For this review, take the finished solid that the model builds, in its own axes (mm). A direction names the side the tool comes from. Round coordinates to 2 decimals unless told otherwise and drop trailing zeros. Write each loop counter-clockwise with the first axis right and the second up, starting at its lowest first coordinate (ties: lowest second). Pieces come first, ordered by that corner, then holes. Notation, with made-up numbers: (25.5, 38.5) -> (32.5, 38.5) arc R25 cw to (32.5, 61.5) -> close; hole circle Ø7 at (-30, -12). An arc over 180 degrees is marked (long way). Answer in a Markdown table with one row per item.
from build123d import *

# Parameters (mm, degrees)
SKETCH_1_W                         = 26.8
SKETCH_1_H                         = 10.5
EXTRUDE_1_DEPTH                    = 8.6
CUT_EXTRUDE_1_DEPTH                = 7
EXTRUDE_START                      = -5
SKETCH_3_W                         = 1
SKETCH_3_H                         = 1
EXTRUDE_2_DEPTH                    = 8.6
CHAMFER_1_SIZE                     = 0.3
SKETCH_4_W                         = 1
SKETCH_4_H                         = 1
EXTRUDE_3_DEPTH                    = 5
PATTERN_LINEAR_1_COUNT             = 7
PATTERN_LINEAR_1_PITCH             = 3.5
CHAMFER_1_OF_PATTERN_LINEAR_1_SIZE = 0.3


with BuildPart() as part:
    # Эскиз1 → Бобышка-Вытянуть1 (new body)
    with BuildSketch(Plane.XY):
        with Locations((0, 5.25)):
            Rectangle(SKETCH_1_W, SKETCH_1_H)
    extrude(amount=EXTRUDE_1_DEPTH)

    # Эскиз2 → Вырез-Вытянуть1 (cut)
    with BuildSketch(Plane.XZ):
        Polygon((-12.4, 6.6), (12.4, 6.6), (12.4, 0.2), (10.2, 0.2), (10.2, 1.8), (-8.6, 1.8), (-8.6, 0.2), (-10.8, 0.2), (-10.8, 1.8), (-12.4, 1.8), align=None)
    extrude(amount=-CUT_EXTRUDE_1_DEPTH, mode=Mode.SUBTRACT)

    # Эскиз3 → Бобышка-Вытянуть2 (add)
    with BuildSketch(Plane(origin=(0, 0, 0), x_dir=(-1, 0, 0), z_dir=(0, 0, -1)).offset(EXTRUDE_START)):
        with Locations((10.5, 9.5)):
            Rectangle(SKETCH_3_W, SKETCH_3_H)
    extrude_2 = extrude(amount=EXTRUDE_2_DEPTH)

    # Фаска1
    chamfer_1_edges = [part.edges().sort_by_distance(p)[0] for p in [
        (-10, 9.5, -3.6),
        (-10.5, 9, -3.6),
        (-11, 9.5, -3.6),
        (-10.5, 10, -3.6),
    ]]
    chamfer(chamfer_1_edges, length=CHAMFER_1_SIZE)

    # Эскиз4 → Бобышка-Вытянуть3 (add)
    with BuildSketch(Plane.XZ.offset(-7)):
        with Locations((-10.5, 4.35)):
            Rectangle(SKETCH_4_W, SKETCH_4_H)
    extrude_3 = extrude(amount=EXTRUDE_3_DEPTH)

    # Линейный массив1: Бобышка-Вытянуть2, Бобышка-Вытянуть3 ×7
    with Locations(*[(i * PATTERN_LINEAR_1_PITCH, 0, 0) for i in range(1, PATTERN_LINEAR_1_COUNT)]):
        add(extrude_2)
        add(extrude_3)

    # Фаска1 of Линейный массив1
    chamfer_1_of_pattern_linear_1_edges = [part.edges().sort_by_distance(p)[0] for p in [
        (-6.5, 9.5, -3.6),
        (-7, 9, -3.6),
        (-7.5, 9.5, -3.6),
        (-7, 10, -3.6),
        (-3, 9.5, -3.6),
        (-3.5, 9, -3.6),
        (-4, 9.5, -3.6),
        (-3.5, 10, -3.6),
        (0.5, 9.5, -3.6),
        (0, 9, -3.6),
        (-0.5, 9.5, -3.6),
        (0, 10, -3.6),
        (4, 9.5, -3.6),
        (3.5, 9, -3.6),
        (3, 9.5, -3.6),
        (3.5, 10, -3.6),
        (7.5, 9.5, -3.6),
        (7, 9, -3.6),
        (6.5, 9.5, -3.6),
        (7, 10, -3.6),
        (11, 9.5, -3.6),
        (10.5, 9, -3.6),
        (10, 9.5, -3.6),
        (10.5, 10, -3.6),
    ]]
    chamfer(chamfer_1_of_pattern_linear_1_edges, length=CHAMFER_1_OF_PATTERN_LINEAR_1_SIZE)


solid = part.part
1) For line 1 (Z direction, x = 10.5, y = 6.75); line 2 (Z direction, x = -5.5, y = 2); line 3 (X direction, y = 4.5, z = 5.5), list the stretches that pass through material, from the lowest coordinate up. Write a range as [from, to].
Solved:
| item | result |
|---|---|
| line 1 | [0, 0.2], [3.85, 4.85], [6.6, 8.6] |
| line 2 | [0, 1.8], [6.6, 8.6] |
| line 3 | [-13.4, -12.4], [12.4, 13.4] |
2) Mouldability with a two-part tool opening along X and no side actions: class faces 1 (the flat face through (10.5, 10, -1.6)), 2 (the flat face through (-7, 5, 3.85)), 3 (the flat face through (11, 9.5, -1.6)), 4 (the flat face through (0, 7, 3)) as pulls with the +X half, pulls with the -X half, needs draft (parallel to the pull), parting line crosses it, or undercut.
Solved:
| item | result |
|---|---|
| face 1 | needs draft |
| face 2 | undercut |
| face 3 | pulls with the +X half |
| face 4 | undercut |
3) Consider section D-D on x = -5.75. State the section outline as (y, z) points, then the cut area to 3 significant figures.
Solved:
| item | result |
|---|---|
| outline | (0, 0) -> (10.5, 0) -> (10.5, 8.6) -> (0, 8.6) -> (0, 6.6) -> (7, 6.6) -> (7, 1.8) -> (0, 1.8) -> close |
| area | 56.7 mm² |
4) Consider section B-B on x = -9.5. State the section outline as (y, z) points.
Solved:
| item | result |
|---|---|
| outline | (0, 0) -> (10.5, 0) -> (10.5, 8.6) -> (0, 8.6) -> (0, 6.6) -> (7, 6.6) -> (7, 0.2) -> (0, 0.2) -> close |
5) Consider section C-C on y = 3. State how many separate pieces and enclosed holes the cut face has, then the cut area to 3 significant figures.
Solved:
| item | result |
|---|---|
| separate pieces | 8 |
| enclosed holes | 1 |
| area | 111 mm² |
6) Clearance check with flat-ended pins moving along their axes: pin 1 Ø3.5 at (x, y) = (4.5, 2) entering from -Z; pin 2 Ø1.1 at (y, z) = (9.5, -1) entering from -X; pin 3 Ø0.5 at (x, z) = (0, -2) entering from -Y; pin 4 Ø2 at (y, z) = (3, -1.5) entering from -X. State where each tip first meets the part, or that it passes through.
Solved:
| item | result |
|---|---|
| pin 1 | z = 0 |
| pin 2 | x = -11 |
| pin 3 | y = 9 |
| pin 4 | through |
7) For faces 5 (the flat face through (-3.5, 9, -1.6)), 6 (the flat face through (0, 5, 8.6)), 7 (the flat face through (7, 5, 4.85)), 8 (the flat face through (-7.5, 9.5, -1.6)), list the 3-axis set-ups (+Z, -Z, +X, -X, +Y, -Y) from which the entire face can be reached by the end or side of a thin tool; tool diameter is ignored.
Solved:
| item | result |
|---|---|
| face 5 | -Z, +X, -X, -Y |
| face 6 | +Z, +X, -X, +Y, -Y |
| face 7 | -Y |
| face 8 | -Z, +Y, -Y |
8) Consider section A-A on z = -2.25. State the section outline as (x, y) points.
Solved:
| item | result |
|---|---|
| outline | (-11, 9) -> (-10, 9) -> (-10, 10) -> (-11, 10) -> close; (-7.5, 9) -> (-6.5, 9) -> (-6.5, 10) -> (-7.5, 10) -> close; (-4, 9) -> (-3, 9) -> (-3, 10) -> (-4, 10) -> close; (-0.5, 9) -> (0.5, 9) -> (0.5, 10) -> (-0.5, 10) -> close; (3, 9) -> (4, 9) -> (4, 10) -> (3, 10) -> close; (6.5, 9) -> (7.5, 9) -> (7.5, 10) -> (6.5, 10) -> close; (10, 9) -> (11, 9) -> (11, 10) -> (10, 10) -> close |
